Design review of the part built by this model. Coordinates are the model's own, in mm. A direction names the side the tool comes from. Give positions to 0.01 mm unless a question says otherwise; leave off trailing zeros. Write each loop counter-clockwise with the first axis right and the second up, starting at its lowest first coordinate (ties: lowest second). Pieces come first, ordered by that corner, then holes. Notation, with made-up numbers: (-13, -1.75) -> (11, -1.75) arc R34 ccw to (11, 31.25) -> close; hole circle Ø3 at (21, 6). An arc over 180 degrees is marked (long way). Put each result on its own line as item: value. Start each with the question number.
from build123d import *

# Parameters (mm, degrees)
SKETCH1_R             = 52.5
BOSS_EXTRUDE1_DEPTH   = 13
SKETCH2_R             = 7.5
CUT_EXTRUDE1_DEPTH    = 76.375725535
SKETCH3_R             = 2.305159733
CUT_EXTRUDE2_DEPTH    = 8.842975
CIRPATTERN1_START     = 4.157024627
CIRPATTERN1_OUTLINE_R = 2.305159733
CIRPATTERN1_DEPTH     = 8.842975373


# Read off the part's stored shape, not the designer's step: CirPattern1
with BuildPart() as part:
    # Sketch1 → Boss-Extrude1 (new body)
    with BuildSketch(Plane(origin=(0, 0, 0), x_dir=(1, 0, 0), z_dir=(0, 1, 0))):
        with Locations(Location((0, 0, 0), (0, 0, 90))):
            Circle(SKETCH1_R)
    extrude(amount=BOSS_EXTRUDE1_DEPTH)

    # Sketch2 → Cut-Extrude1 (cut, through all)
    with BuildSketch(Plane(origin=(0, 0, 0), x_dir=(1, 0, 0), z_dir=(0, 1, 0))):
        with Locations(Location((0, 0, 0), (0, 0, 90))):
            Circle(SKETCH2_R)
    extrude(amount=CUT_EXTRUDE1_DEPTH, mode=Mode.SUBTRACT)

    # Sketch3 → Cut-Extrude2 (cut)
    with BuildSketch(Plane(origin=(0, 13, 0), x_dir=(1, 0, 0), z_dir=(0, 1, 0))):
        with Locations(Location((-21.422945149, 0, 0), (0, 0, 270))):
            Circle(SKETCH3_R)
    extrude(amount=-CUT_EXTRUDE2_DEPTH, mode=Mode.SUBTRACT)

    # CirPattern1 outline → CirPattern1 (cut)
    with BuildSketch(Plane(origin=(0, 0, 0), x_dir=(1, 0, 0), z_dir=(0, 1, 0)).offset(CIRPATTERN1_START)):
        with Locations((0, 21.422945149)):
            Circle(CIRPATTERN1_OUTLINE_R)
        with Locations((21.422945149, 0)):
            Circle(CIRPATTERN1_OUTLINE_R)
        with Locations((0, -21.422945149)):
            Circle(CIRPATTERN1_OUTLINE_R)
    extrude(amount=CIRPATTERN1_DEPTH, mode=Mode.SUBTRACT)


solid = part.part
Q1. To check wall thickness, follow probe 1 along X at (y, z) = (7.25, 0); probe 2 along X at (y, z) = (3, 0); probe 3 along X at (y, z) = (5, 22). State the ranges of each line that lie inside material, in increasing order. Write a range as from..to.
Q2. Take a section at A-A on z = 0. Give the boundary of the cut face in (x, y), then the cut area to 3 significant figures.
Q3. Machinability: for faces 5 (the face through (-1, 13, -11)), 6 (the face through (-23.673, 8.64, -0.5)), which of the approach directions +Z, -Z, +X, -X, +Y, -Y give a long, thin tool a straight path to every point of the face, cutting with its end or side? Answer none if there is none.
Q4. Take a section at C-C on y = 10.5. Give the boundary of the cut face in (x, z), then the cut area to 3 significant figures.
Q5. Take a section at B-B on x = 0. Give the boundary of the cut face in (y, z), then the cut area to 3 significant figures.
Q6. Take a section at D-D on x = 43. Give the boundary of the cut face in (y, z), then the cut area to 3 significant figures.
Q7. Mouldability with a two-part tool opening along Z and no side actions: class faces 1 (the face through (-0.33, 6.409, 7.493)), 2 (the face through (-15.77, 6.409, -50.076)), 3 (the face through (11, 0, 1)), 4 (the face through (0, 4.157, -21)) as +Z half, -Z half, draft (parallel to the pull), parting line (faces both ways), or undercut.
Q8. For pin 1 (12 mm diameter, centred on x = 0, z = 0, fed in from -Y); pin 2 (3 mm diameter, centred on x = 21.42, z = 0, fed in from +Y); pin 3 (5 mm diameter, centred on y = 10, z = 22, fed in from +X); pin 4 (7.5 mm diameter, centred on x = 0, z = -21.42, fed in from +Y), all flat-tipped, find the tip position at first contact; note any pin that passes through.
Result:
1. probe 1: x = -52.5..-23.73, -19.12..-7.5, 7.5..19.12, 23.73..52.5
1. probe 2: x = -52.5..-7.5, 7.5..52.5
1. probe 3: x = -47.67..-2.23, 2.23..47.67
2. outline: (-52.5, 0) -> (-7.5, 0) -> (-7.5, 13) -> (-19.12, 13) -> (-19.12, 4.16) -> (-23.73, 4.16) -> (-23.73, 13) -> (-52.5, 13) -> close; (7.5, 0) -> (52.5, 0) -> (52.5, 13) -> (23.73, 13) -> (23.73, 4.16) -> (19.12, 4.16) -> (19.12, 13) -> (7.5, 13) -> close
2. area: 1,090 mm^2
3. face 5: +Z, -Z, +X, -X, +Y
3. face 6: +Y
4. outline: circle Ø105 at (0, 0); hole circle Ø4.61 at (-21.42, 0); hole circle Ø15 at (0, 0); hole circle Ø4.61 at (0, -21.42); hole circle Ø4.61 at (0, 21.42); hole circle Ø4.61 at (21.42, 0)
4. area: 8,420 mm^2
5. outline: (0, -52.5) -> (13, -52.5) -> (13, -23.73) -> (4.16, -23.73) -> (4.16, -19.12) -> (13, -19.12) -> (13, -7.5) -> (0, -7.5) -> close; (0, 7.5) -> (13, 7.5) -> (13, 19.12) -> (4.16, 19.12) -> (4.16, 23.73) -> (13, 23.73) -> (13, 52.5) -> (0, 52.5) -> close
5. area: 1,090 mm^2
6. outline: (0, -30.12) -> (13, -30.12) -> (13, 30.12) -> (0, 30.12) -> close
6. area: 783 mm^2
7. face 1: undercut
7. face 2: parting line
7. face 3: draft
7. face 4: undercut
8. pin 1: passes through
8. pin 2: stops at y = 4.16
8. pin 3: stops at x = 48.74
8. pin 4: stops at y = 13
